The drawing under review shows one solid part. Ordinate dimensions are in mm from its lowest x, y, z. A direction names the side the tool comes from. Give positions to 0.01 mm unless a question says otherwise; leave off trailing zeros. Order: outer loops, then holes, each group sorted by start corner. A loop starts at its lowest first (then second) coordinate and runs counter-clockwise, first axis right, second up. Notation, with made-up numbers: (-17, 21) - (0, 21) arc R19 ccw to (0, 55) - close; hole circle Ø3 at (28.25, 50.25). An arc over 180 degrees is marked (long way). Write item = value, one per line. Start each with the question number.
1. For P1, Ø1, axis at y = 3, z = 9, coming from the +X side; P2, Ø1, axis at x = 7, z = 5, coming from the -Y side, all flat-tipped, find the tip position at first contact; note any pin that passes through.
2. We need section D-D, the plane x = 35. Give the boundary of the cut face in (y, z), and give its area (3 significant figures).
3. Wall thickness on probe 1 along Y at (x, z) = (46, 22.5); probe 2 along Z at (x, y) = (18, 2.75); probe 3 along X at (y, z) = (0.75, 5.5): over which ranges is each line inside the solid? List them lowest first.
4. Mouldability with a two-part tool opening along Y and no side actions: class the marked faces 1, 2 and 3 as pulls with the +Y half, pulls with the -Y half, needs draft (parallel to the pull), parting line crosses it, or undercut.
5. We need section B-B, the plane y = 2.5. Give the boundary of the cut face in (x, z).
6. We need section A-A, the plane x = 46. Give the boundary of the cut face in (y, z).
7. We need section C-C, the plane y = 5.75. Give the boundary of the cut face in (x, z).
8. Machinability: for the marked faces 4 and 5, which of the approach directions +Z, -Z, +X, -X, +Y, -Y give a long, thin tool a straight path to every point of the face, cutting with its end or side? Answer none if there is none.
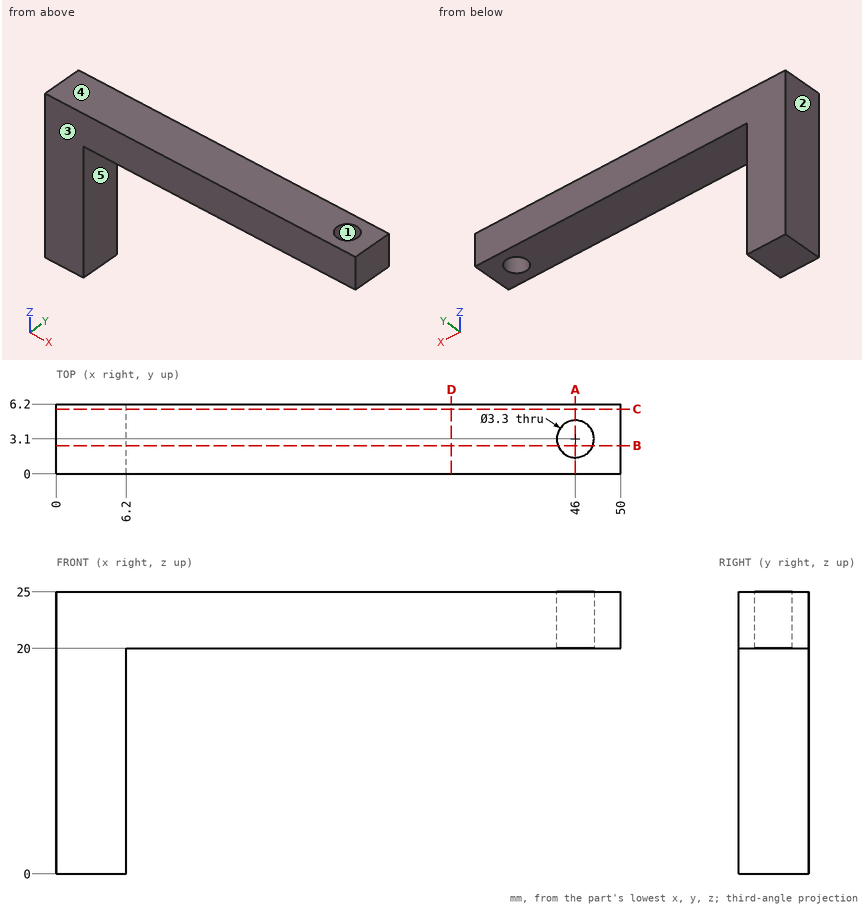
Model answer:
q1.P1 = 6.2
q1.P2 = through
q2.outline = (0, 20) - (6.2, 20) - (6.2, 25) - (0, 25) - close
q2.area = 31.0 mm2
q3.probe_1 = 0 to 1.45, 4.75 to 6.2
q3.probe_2 = 20 to 25
q3.probe_3 = 0 to 6.2
q4.face_1 = undercut
q4.face_2 = needs draft
q4.face_3 = pulls with the -Y half
q5.outline = (0, 0) - (6.2, 0) - (6.2, 20) - (44.46, 20) - (44.46, 25) - (0, 25) - close; (47.54, 20) - (50, 20) - (50, 25) - (47.54, 25) - close
q6.outline = (0, 20) - (1.45, 20) - (1.45, 25) - (0, 25) - close; (4.75, 20) - (6.2, 20) - (6.2, 25) - (4.75, 25) - close
q7.outline = (0, 0) - (6.2, 0) - (6.2, 20) - (50, 20) - (50, 25) - (0, 25) - close
q8.face_4 = +Z, +X, -X, +Y, -Y
q8.face_5 = -Z, +X, +Y, -Y
